from build123d import *

# Parameters (mm, degrees)
F2_R      = 1.169
F2_R_2    = 1.0196666667
F2_R_3    = 1.0213333333
F2_R_4    = 0.55
F2_R_5    = 0.8
F2_R_6    = 0.869
F2_R_7    = 0.5
F2_R_8    = 0.675
F3_DEPTH  = 6.501
F4_R      = 1
F5_R      = 0.2
F6_SIZE   = 0.2
F8_DEPTH  = 0.5
F9_R      = 0.675
F10_DEPTH = 10.701
F11_R     = 0.92
F11_R_2   = 0.675
F12_DEPTH = 1.2
F13_SCALE = 3


with BuildPart() as f1:
    # F0 (on Front) → F1 (revolve)
    with BuildSketch(Plane.XZ):
        Polygon((3.25, 5.2), (3.25, 0), (6.5, 0), (6.5, 4.7), (21.3536666667, 4.7), (21.3536666667, 6.7), (3.9775, 6.7), (3.9775, 7.5), (3, 7.5), (3, 8.35), (3.9775, 8.35), (3.9775, 11.2), (1.5213333333, 11.2), (1.5213333333, 5.2), align=None)
    revolve(axis=Axis((0, 0, 5.6), (0, 0, 1)))

    # F2 (on face) → F3 (cut, through all)
    with BuildSketch(Plane(origin=(0, 0, 4.7), x_dir=(1, 0, 0), z_dir=(0, 0, -1))):
        with Locations((19.5, 0)):
            Circle(F2_R)
        with Locations((18.3240061053, -6.6693927949)):
            Circle(F2_R)
        with Locations((14.9378666408, -12.5343583889)):
            Circle(F2_R)
        with Locations((9.75, -16.8874953738)):
            Circle(F2_R)
        with Locations((3.3861394645, -19.2037511837)):
            Circle(F2_R)
        with Locations((-3.3861394645, -19.2037511837)):
            Circle(F2_R)
        with Locations((-9.75, -16.8874953738)):
            Circle(F2_R)
        with Locations((-14.9378666408, -12.5343583889)):
            Circle(F2_R)
        with Locations((-17.6164932368, -7.1175252749)):
            Circle(F2_R_2)
        with Locations((11.6913429511, 6.75)):
            Circle(F2_R_3)
        with Locations((8.6776327308, 10.3415999821)):
            Circle(F2_R_3)
        with Locations((12.6858503806, -4.6172719349)):
            Circle(F2_R_3)
        with Locations((13.5, 0)):
            Circle(F2_R_3)
        with Locations((10.3415999821, -8.6776327308)):
            Circle(F2_R_3)
        with Locations((6.75, -11.6913429511)):
            Circle(F2_R_3)
        with Locations((2.3442503985, -13.2949046657)):
            Circle(F2_R_3)
        with Locations((-2.3442503985, -13.2949046657)):
            Circle(F2_R_3)
        with Locations((-6.75, -11.6913429511)):
            Circle(F2_R_3)
        with Locations((-10.3415999821, -8.6776327308)):
            Circle(F2_R_3)
        with Locations((-12.6858503806, -4.6172719349)):
            Circle(F2_R_3)
        with Locations((-13.5, 0)):
            Circle(F2_R_3)
        with Locations((-12.6858503806, 4.6172719349)):
            Circle(F2_R_3)
        with Locations((-8.6776327308, 10.3415999821)):
            Circle(F2_R_3)
        with Locations((-4.6172719349, 12.6858503806)):
            Circle(F2_R_3)
        with Locations((0, 13.5)):
            Circle(F2_R_3)
        with Locations((4.6172719349, 12.6858503806)):
            Circle(F2_R_3)
        with Locations((18.7113473072, -3.2993153757)):
            Circle(F2_R_4)
        with Locations((12.212964584, -14.5548444193)):
            Circle(F2_R_4)
        with Locations((0, -19)):
            Circle(F2_R_4)
        with Locations((-12.212964584, -14.5548444193)):
            Circle(F2_R_4)
        with Locations((6.4983827232, -17.8541597949)):
            Circle(F2_R_5)
        with Locations((17.6164932368, 7.1175252749)):
            Circle(F2_R_2)
        with Locations((13.5, 11.2)):
            Circle(F2_R_6)
        with Locations((11.1842488695, 9.3846991014)):
            Circle(F2_R_7)
        with Locations((-6.4983827232, 17.8541597949)):
            Circle(F2_R_5)
        with Locations((-12.7134815208, 14.1197516841)):
            Circle(F2_R_2)
        with Locations((-17.2341356777, 3.0388431092)):
            Circle(F2_R_8)
        with Locations((-14.3341356777, 2.5274948651)):
            Circle(F2_R_7)
        with BuildLine():
            Line((6.1013408583, 20.4634483859), (5.7339118404, 19.3326181465))
            ThreePointArc((5.7339118404, 19.3326181465), (5.4788713103, 16.8622320339), (6.7245957116, 19.010725444))
            Line((6.7245957116, 19.010725444), (7.0920247294, 20.1415556834))
            ThreePointArc((7.0920247294, 20.1415556834), (6.5986458922, 20.3085438301), (6.1013408583, 20.4634483859))
        make_face()
    extrude(amount=-F3_DEPTH, mode=Mode.SUBTRACT)

    # F4
    f4_edges = [f1.edges().sort_by_distance(p)[0] for p in [
        (-6.5, 0, 4.7),
    ]]
    fillet(f4_edges, radius=F4_R)

    # F5
    f5_edges = [f1.edges().sort_by_distance(p)[0] for p in [
        (-3.9775, 0, 6.7),
    ]]
    fillet(f5_edges, radius=F5_R)

    # F6
    f6_edges = [f1.edges().sort_by_distance(p)[0] for p in [
        (-3.9775, 0, 11.2),
    ]]
    chamfer(f6_edges, length=F6_SIZE)

    # F7 (on face) → F8 (cut)
    with BuildSketch(Plane(origin=(0, 0, 0), x_dir=(1, 0, 0), z_dir=(0, 0, -1))):
        with BuildLine():
            ThreePointArc((-5.8803865992, 2.7696666667), (-6.5, 0), (-5.8803865992, -2.7696666667))
            Line((-5.8803865992, -2.7696666667), (-1.7004254043, -2.7696666667))
            ThreePointArc((-1.7004254043, -2.7696666667), (-3.25, 0), (-1.7004254043, 2.7696666667))
            Line((-1.7004254043, 2.7696666667), (-5.8803865992, 2.7696666667))
        make_face()
        with BuildLine():
            Line((1.7004254043, -2.7696666667), (5.8803865992, -2.7696666667))
            ThreePointArc((5.8803865992, -2.7696666667), (6.3432055341, -1.419064323), (6.5, 0))
            ThreePointArc((6.5, 0), (6.3432055341, 1.419064323), (5.8803865992, 2.7696666667))
            Line((5.8803865992, 2.7696666667), (1.7004254043, 2.7696666667))
            ThreePointArc((1.7004254043, 2.7696666667), (2.8362724273, 1.5868392225), (3.25, 0))
            ThreePointArc((3.25, 0), (2.8362724273, -1.5868392225), (1.7004254043, -2.7696666667))
        make_face()
    extrude(amount=-F8_DEPTH, mode=Mode.SUBTRACT)

    # F9 (on face) → F10 (cut, through all)
    with BuildSketch(Plane(origin=(0, 0, 0.5), x_dir=(1, 0, 0), z_dir=(0, 0, -1))):
        with Locations((-4.9, 0)):
            Circle(F9_R)
    extrude(amount=-F10_DEPTH, mode=Mode.SUBTRACT)

    # F11 (on face) → F12 (cut)
    with BuildSketch(Plane(origin=(0, 0, 0.5), x_dir=(1, 0, 0), z_dir=(0, 0, -1))):
        with Locations((-4.9, 0)):
            Circle(F11_R)
        with Locations((-4.9, 0)):
            Circle(F11_R_2, mode=Mode.SUBTRACT)
        with Locations((-4.9, 0)):
            Circle(F11_R_2)
    extrude(amount=-F12_DEPTH, mode=Mode.SUBTRACT)


with BuildPart() as f1_1:
    # F13: moved
    add(f1.part.scale(F13_SCALE))


solid = f1_1.part
Could you check a few things on this model? Use its own coordinates, in mm. A direction names the side the tool comes from. Give positions to 0.01 mm unless a question says otherwise; leave off trailing zeros. Order: outer loops, then holes, each group sorted by start corner. A loop starts at its lowest first (then second) coordinate and runs counter-clockwise, first axis right, second up.
1. Suppose I cut it at A-A (x = 0). Give the number of separate pieces and of enclosed holes in the cut face, plus the area to 3 significant figures.
2. Suppose I cut it at B-B (z = 3.5). List the corners of the cut face in (x, y) for me, plus the area to 3 significant figures.
3. We'd pull the mould along Z, two halves only. Please class faces 1 (the flat face through (-2, 9, 25.05)), 2 (the flat face through (-16, -2, 5.1)), 3 (the cylindrical face through (-41.12, -13.99, 17.06)): pulls with the +Z half, pulls with the -Z half, needs draft (parallel to the pull), parting line crosses it, or undercut.
4. Suppose I cut it at C-C (z = 27). List the corners of the cut face in (x, y) for me (1 decimal), plus the area to 3 significant figures.
5. For faces 4 (the cylindrical face through (-53.51, 24.34, 17.06)), 5 (the cylindrical face through (-12.067, -0.829, 3.275)), which set-ups out of +Z, -Z, +X, -X, +Y, -Y let a thin tool reach every point of the face, with its end or its side?
6. I need wall thicknesses on L1, parallel to Y at x = 0, z = 17.65; L2, parallel to Z at x = -47.5, y = 10; L3, parallel to X at y = 24, z = 16. Which ranges of each line are inside material? Lowest first, please.
7. Will these pins go through, and if not, where does the flat tip stop? P1, Ø6, axis at x = -37.5, z = 12.5, coming from the -Y side; P2, Ø8, axis at y = 21, z = 16, coming from the +X side; P3, Ø1.2, axis at x = 9.5, z = 0.5, coming from the +Y side; P4, Ø15.5, axis at x = 4, y = 4.5, coming from the -Z side.
Solved:
1. separate pieces: 4
1. enclosed holes: 0
1. area: 1,100 mm2
2. outline: circle Ø39 at (0, 0); hole circle Ø5.52 at (-14.7, 0); hole circle Ø19.5 at (0, 0)
2. area: 872 mm2
3. face 1: undercut
3. face 2: pulls with the -Z half
3. face 3: needs draft
4. outline: circle Ø23.9 at (0, 0); hole circle Ø9.1 at (0, 0)
4. area: 382 mm2
5. face 4: +Z, -Z
5. face 5: -Z
6. L1: y = -64.06 to -43.56, -37.44 to -4.56, 4.56 to 55.35, 58.65 to 64.06
6. L2: z = 14.1 to 20.1
6. L3: x = -59.4 to -54.38, -51.32 to -33.32, -28.73 to 28.73, 33.32 to 59.4
7. P1: stops at y = -53.68
7. P2: stops at x = 61.76
7. P3: stops at y = 17.35
7. P4: stops at z = 0
